from build123d import *

# Parameters (mm, degrees)
SKETCH_1_R          = 3
SKETCH_1_R_2        = 10
SKETCH_1_R_3        = 1
EXTRUDE_1_DEPTH     = 5
SKETCH_2_R          = 12.5
SKETCH_2_R_2        = 10
EXTRUDE_2_DEPTH     = 70
SKETCH_3_R          = 12.5
EXTRUDE_3_DEPTH     = 15
SKETCH_4_R          = 4
CUT_EXTRUDE_1_DEPTH = 96.436281211
SKETCH_5_R          = 7.5
CUT_EXTRUDE_2_DEPTH = 12
SKETCH_6_R          = 9.5
CUT_EXTRUDE_3_DEPTH = 3


with BuildPart() as part:
    # Эскиз1 → Бобышка-Вытянуть1 (new body)
    with BuildSketch(Plane(origin=(0, 0, 0), x_dir=(1, 0, 0), z_dir=(0, 1, 0))):
        with BuildLine():
            Line((-22.5, 4.130728704), (0, 14.130728704))
            Line((0, 14.130728704), (22.5, 4.130728704))
            ThreePointArc((22.5, 4.130728704), (27.5, -0.869271296), (22.5, -5.869271296))
            Line((22.5, -5.869271296), (0, -15.869271296))
            Line((0, -15.869271296), (-22.5, -5.869271296))
            ThreePointArc((-22.5, -5.869271296), (-27.5, -0.869271296), (-22.5, 4.130728704))
        make_face()
        with Locations(Location((-22.5, -0.869271296, 0), (0, 0, 270))):
            Circle(SKETCH_1_R, mode=Mode.SUBTRACT)
        with Locations(Location((0, -0.869271296, 0), (0, 0, 270))):
            Circle(SKETCH_1_R_2, mode=Mode.SUBTRACT)
        with Locations(Location((22.5, -0.869271296, 0), (0, 0, 270))):
            Circle(SKETCH_1_R, mode=Mode.SUBTRACT)
        with Locations(Location((-16.5, -0.869271296, 0), (0, 0, 270))):
            Circle(SKETCH_1_R_3, mode=Mode.SUBTRACT)
        with Locations(Location((16.5, -0.869271296, 0), (0, 0, 270))):
            Circle(SKETCH_1_R_3, mode=Mode.SUBTRACT)
    extrude(amount=EXTRUDE_1_DEPTH)

    # Эскиз2 → Бобышка-Вытянуть2 (add)
    with BuildSketch(Plane(origin=(0, 5, 0), x_dir=(1, 0, 0), z_dir=(0, 1, 0))):
        with Locations(Location((0, -0.869271296, 0), (0, 0, 270))):
            Circle(SKETCH_2_R)
        with Locations(Location((0, -0.869271296, 0), (0, 0, 270))):
            Circle(SKETCH_2_R_2, mode=Mode.SUBTRACT)
    extrude(amount=EXTRUDE_2_DEPTH)

    # Эскиз3 → Бобышка-Вытянуть3 (add)
    with BuildSketch(Plane(origin=(0, 75, 0), x_dir=(1, 0, 0), z_dir=(0, 1, 0))):
        with Locations(Location((0, -0.869271296, 0), (0, 0, 270))):
            Circle(SKETCH_3_R)
    extrude(amount=EXTRUDE_3_DEPTH)

    # Эскиз4 → Вырез-Вытянуть1 (cut, through all)
    with BuildSketch(Plane(origin=(0, 90, 0), x_dir=(1, 0, 0), z_dir=(0, 1, 0))):
        with Locations(Location((0, -0.869271296, 0), (0, 0, 270))):
            Circle(SKETCH_4_R)
    extrude(amount=-CUT_EXTRUDE_1_DEPTH, mode=Mode.SUBTRACT)

    # Эскиз5 → Вырез-Вытянуть2 (cut)
    with BuildSketch(Plane(origin=(0, 90, 0), x_dir=(1, 0, 0), z_dir=(0, 1, 0))):
        with Locations(Location((0, -0.869271296, 0), (0, 0, 270))):
            Circle(SKETCH_5_R)
    extrude(amount=-CUT_EXTRUDE_2_DEPTH, mode=Mode.SUBTRACT)

    # Эскиз6 → Вырез-Вытянуть3 (cut)
    with BuildSketch(Plane(origin=(0, 90, 0), x_dir=(1, 0, 0), z_dir=(0, 1, 0))):
        with Locations(Location((0, -0.869271296, 0), (0, 0, 270))):
            Circle(SKETCH_6_R)
    extrude(amount=-CUT_EXTRUDE_3_DEPTH, mode=Mode.SUBTRACT)


solid = part.part
Verification items for the finished model (mm, model axes). A direction names the side the tool comes from. Coordinates: 2 decimals unless noted, no trailing zeros. Write each loop counter-clockwise with the first axis right and the second up, starting at its lowest first coordinate (ties: lowest second). Pieces come first, ordered by that corner, then holes. Notation, with made-up numbers: M 49,76.5 L 88,76.5 A23 cw 88,92.5 Z; hole C -26,-21 d1. An arc over 180 degrees is marked long. One line per question, with ' | ' between items.
1) Access from +Z, -Z, +X, -X, +Y, -Y to the whole of each face (thin tool, end or side, straight path). Record for faces 4 (the face through (27.5, 2.5, 0.8)), 5 (the face through (3, 87, 8)), 6 (the face through (-4.3, 75, 0.7)).
Solutions:
face 4: +X, +Y, -Y | face 5: +Y | face 6: -Y
2) Material ranges on L1, parallel to Y at x = -1.5, z = 7; L2, parallel to X at y = 9.5, z = 9.5; L3, parallel to Z at x = -9, y = 68, recorded low to high.
Solutions:
L1: 75 to 78 | L2: -9.04 to -5.05, 5.05 to 9.04 | L3: -7.81 to -3.49, 5.23 to 9.54
3) Sectioned sample at A-A on x = 1. Record the cut outline in (y, z).
Solutions:
outline: M 0,-13.69 L 5,-13.69 L 5,-11.59 L 90,-11.59 L 90,-8.58 L 87,-8.58 L 87,-6.56 L 78,-6.56 L 78,-3 L 75,-3 L 75,-9.08 L 0,-9.08 Z; M 0,10.82 L 75,10.82 L 75,4.74 L 78,4.74 L 78,8.3 L 87,8.3 L 87,10.32 L 90,10.32 L 90,13.33 L 5,13.33 L 5,15.42 L 0,15.42 Z
4) Depth check by flat-ended pin: pin 1 Ø9 at (x, z) = (0, 0.87) entering from -Y; pin 2 Ø16.5 at (x, z) = (-0.5, 0.5) entering from +Y; pin 3 Ø1.8 at (x, z) = (16.5, 0.87) entering from +Y; pin 4 Ø1 at (x, z) = (0.5, 6) entering from +Y. Enter the tip coordinate at first touch or a pass-through.
Solutions:
pin 1: y = 75 | pin 2: y = 87 | pin 3: through | pin 4: y = 78
5) Sectioned sample at D-D on z = 12. Record the cut outline in (x, y).
Solutions:
outline: M -8.71,0 L 8.71,0 L 8.71,5 L 5.69,5 L 5.69,90 L -5.69,90 L -5.69,5 L -8.71,5 Z
6) Sectioned sample at B-B on y = 67. Record the cut outline in (x, z), then the cut area to 3 significant figures.
Solutions:
outline: C 0,0.87 d25; hole C 0,0.87 d20 | area: 177 mm^2
7) Sectioned sample at C-C on x = -16.5. Record the cut outline in (y, z), then the cut area to 3 significant figures.
Solutions:
outline: M 0,-6.8 L 5,-6.8 L 5,-0.13 L 0,-0.13 Z; M 0,1.87 L 5,1.87 L 5,8.54 L 0,8.54 Z | area: 66.7 mm^2
8) Release check for a two-part mould opening along X. For faces 1 (the face through (9.3, 90, 3.6)), 2 (the face through (-27.5, 2.5, 1)), 3 (the face through (3, 36.98, 10.41)) record: +X half, -X half, draft (parallel to the pull), parting line (faces both ways), or undercut.
Solutions:
face 1: draft | face 2: -X half | face 3: undercut
